Autodesk Inventor part; units mm, degrees
ref_plane "Work Plane1" through (0, -9.525, 0) normal (0, -1, 0) x (1, 0, 0)
ref_plane "Work Plane2" through (0, 9.525, 0) normal (0, 1, 0) x (1, 0, 0)
ref_plane "YZ Plane" through (0, 0, 0) normal (1, 0, 0) x (0, 1, 0)
sketch "Sketch1" plane through (0, 0, 0) normal (0, 0, 1) x (1, 0, 0)
  line L0 (-3.3274, -3.3274) -> (3.3274, -3.3274)
  line L1 (3.3274, -3.3274) -> (3.3274, 3.3274)
  line L2 (3.3274, 3.3274) -> (-3.3274, 3.3274)
  line L3 (-3.3274, 3.3274) -> (-3.3274, -3.3274)
  line L4 (-3.3274, -3.3274) -> (3.3274, 3.3274) construction
  line L5 (3.3274, -3.3274) -> (-3.3274, 3.3274) construction
  circle A0 centre (0, 0) radius 9.525
  line L6 (-4.5974, 0.3969) -> (11.7358, 0.3969)
  line L7 (11.7358, 0.3969) -> (11.7358, -0.3969)
  line L8 (11.7358, -0.3969) -> (-4.5974, -0.3969)
  line L9 (-4.5974, -0.3969) -> (-4.5974, 0.3969)
  point P0 (-4.5974, 0)
  point P1 (-3.3274, -0.3969)
  point P2 (-3.3274, 0.3969)
  point P3 (3.3274, 0.3969)
  point P4 (9.5167, 0.3969)
  point P5 (9.5167, -0.3969)
  point P6 (3.3274, -0.3969)
  dimension "d0" = 6.6548
  dimension "d1" = 6.6548
  dimension "d2" = 19.05
  dimension "d3" = 0.7937
  dimension "d4" = 1.27
extrude "Extrusion1" add sketch "Sketch1" along normal blind 63.5 contours L0 L1 L8 A0 L6 L2 L3 L9
sketch "Sketch2" plane through (3.3274, 0.3969, 0) normal (0, -1, 0) x (1, 0, 0)
  circle A0 centre (3.0947, 57.15) radius 2.286
  line L0 (0, 63.5) -> (6.1893, 63.5)
  line L1 (6.1893, 0) -> (6.1893, 63.5)
  line L2 (6.1893, 31.75) -> (0, 31.75)
  line L3 (0, 0) -> (0, 63.5)
  circle A1 centre (3.0947, 6.35) radius 2.286
  point P0 (-3.3274, 0)
  point P1 (3.0947, 63.5)
  dimension "d7" = 4.572
  dimension "d8" = 6.35
extrude "Extrusion2" cut sketch "Sketch2" along normal mid plane 63.5 contours A0 | A1
ref_plane "Work Plane1" through (0, -9.525, 0) normal (0, -1, 0) x (1, 0, 0)
ref_plane "Work Plane2" through (0, 9.525, 0) normal (0, 1, 0) x (1, 0, 0)
sketch "Sketch3" plane through (0, -9.525, 0) normal (0, -1, 0) x (1, 0, 0)
  circle A0 centre (6.4221, 6.35) radius 2.286
  circle A1 centre (6.4221, 6.35) radius 4.1275
  line L0 (6.4221, 10.4775) -> (9.5167, 10.4775)
  line L1 (9.5167, 0) -> (9.5167, 63.5)
  line L2 (6.4221, 2.2225) -> (9.5167, 2.2225)
  line L3 (-9.525, 0) -> (-9.525, 63.5)
  line L4 (-9.525, 31.75) -> (9.5167, 31.75)
  circle A2 centre (6.4221, 57.15) radius 4.1275
  line L5 (6.4221, 53.0225) -> (9.5167, 53.0225)
  line L6 (6.4221, 61.2775) -> (9.5167, 61.2775)
  point P0 (0, 0)
  dimension "d11" = 8.255
extrude "Extrusion3" cut sketch "Sketch3" against normal blind 5.715 contours A1 L1 | L0 L1 A1 | A1 L1 L2 | L5 A2 L1 | A2 L1 | A2 L6 L1 picked at (9.2472, 6.35) picked at (7.5728, 58.1798)
sketch "Sketch4" plane through (0, 9.525, 0) normal (0, 1, 0) x (1, 0, 0)
  circle A0 centre (6.4221, -6.35) radius 2.286
  arc A1 (6.4221, -2.2225) -> (6.4221, -10.4775) centre (6.4221, -6.35) ccw
  line L0 (0.9228, -6.35) -> (3.6724, -1.5875)
  line L1 (3.6724, -1.5875) -> (9.1717, -1.5875)
  line L2 (9.1717, -1.5875) -> (11.9213, -6.35)
  line L3 (11.9213, -6.35) -> (9.1717, -11.1125)
  line L4 (9.1717, -11.1125) -> (3.6724, -11.1125)
  line L5 (3.6724, -11.1125) -> (0.9228, -6.35)
  line L6 (-9.525, 0) -> (-9.525, -63.5)
  line L7 (-9.525, -31.75) -> (9.525, -31.75)
  line L8 (9.1717, -11.1125) -> (11.7374, -11.1125)
  line L9 (11.7374, -11.1125) -> (11.7374, -1.5875)
  line L10 (11.7374, -1.5875) -> (9.1717, -1.5875)
  line L11 (0.9228, -57.15) -> (3.6724, -61.9125)
  line L12 (3.6724, -61.9125) -> (9.1717, -61.9125)
  line L13 (9.1717, -61.9125) -> (11.9213, -57.15)
  line L14 (11.9213, -57.15) -> (9.1717, -52.3875)
  line L15 (9.1717, -52.3875) -> (3.6724, -52.3875)
  line L16 (3.6724, -52.3875) -> (0.9228, -57.15)
  line L17 (9.1717, -52.3875) -> (11.7374, -52.3875)
  line L18 (11.7374, -52.3875) -> (11.7374, -61.9125)
  line L19 (11.7374, -61.9125) -> (9.1717, -61.9125)
  point P0 (0, 0)
  point P1 (11.7374, -6.6685)
  point P2 (11.7374, -6.0315)
  dimension "d16" = 9.525
extrude "Extrusion4" cut sketch "Sketch4" against normal blind 6.096 contours A0 | L0 L1 L2 L9 L3 L4 L5 | L10 L9 L2 | L3 L9 L8 | L16 L15 L14 L18 L13 L12 L11 | L13 L18 L19 | L17 L18 L14
sketch "Sketch5" plane through (0, 0, 63.5) normal (0, 0, 1) x (1, 0, 0)
  line L0 (4.1361, -3.81) -> (8.7081, -3.81)
  arc A0 (9.5167, 0.3969) -> (9.5167, -0.3969) centre (0, 0) ccw
  line L1 (8.1359, -4.953) -> (-8.1359, -4.953)
  arc A1 (-8.1359, -4.953) -> (8.1359, -4.953) centre (0, 0) ccw
  dimension "d17" = 1.143
extrude "Extrusion5" cut sketch "Sketch5" against normal up to surface (63.5 mm away)
fillet "Fillet1" radius 3.175 1 edges at (-8.1359, -4.953, 31.75)
fillet "Fillet2" radius 2.54 3 edges at (8.1359, -4.953, 31.75) (8.1359, -4.953, 62.3888) (8.1359, -4.953, 1.1112)
properties part number "AxleBar"
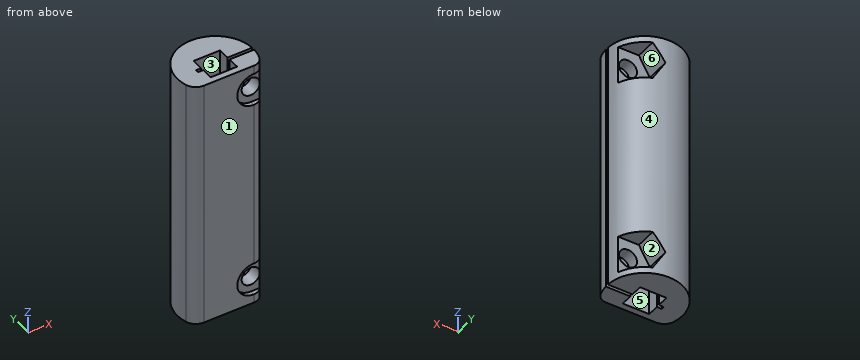
The listing builds one solid part. Answer for the finished solid, in the listing's coordinates (mm). Face numbers are marked on the shaded views. A direction names the side the tool comes from. Round coordinates to 2 decimals unless told otherwise and drop trailing zeros. Order: outer loops, then holes, each group sorted by start corner. A loop starts at its lowest first (then second) coordinate and runs counter-clockwise, first axis right, second up. Notation, with made-up numbers: (9.25, -18) -> (53.25, -18) arc R11 ccw to (53.25, -7) -> close; hole circle Ø5 at (3.25, 39). An arc over 180 degrees is marked (long way). One line per item, written item: value.
Item 1: For a pull along X with two mould halves and no side action, classify the marked faces 3, 4, 5 and 6 as released by +X, released by -X, zero draft, split by the parting line, or undercut.
Taken from the geometry:
face 3: undercut
face 4: split by the parting line
face 5: undercut
face 6: released by +X
Item 2: Find section A-A, the plane x = 0. Give the vertices of the cut face in (y, z) (3 decimals), then the cut area to 3 significant figures.
Taken from the geometry:
outline: (-4.953, 0) -> (-3.327, 0) -> (-3.327, 63.5) -> (-4.953, 63.5) -> close; (3.327, 0) -> (9.525, 0) -> (9.525, 63.5) -> (3.327, 63.5) -> close
area: 497 mm2
Item 3: For the marked faces 1 and 2, determine the directions among +Z, -Z, +X, -X, +Y, -Y from which every point of the face is accessible in a straight line to the end or side of a thin tool.
Taken from the geometry:
face 1: +Z, -Z, +X, -X, -Y
face 2: +X, +Y
Item 4: Straight lines are drawn through the part: L1, parallel to Z at x = 6.5, y = 5.25; L2, parallel to Z at x = 6.5, y = 2.5; L3, parallel to Y at x = 1, z = 20. For each, find the intervals that lie inside material, in ascending order.
Taken from the geometry:
L1: z = 0 to 1.59, 11.11 to 52.39, 61.91 to 63.5
L2: z = 0 to 4.07, 8.63 to 54.87, 59.43 to 63.5
L3: y = -4.95 to -3.33, 3.33 to 9.47
Item 5: Given P1, Ø3, axis at y = 5.5, z = 18, coming from the -X side; P2, Ø3, axis at x = -5, z = 44, coming from the +Y side; P3, Ø3, axis at x = 7, z = 44.5, coming from the +Y side; P4, Ø2.5, axis at x = 6.42, z = 57.15, coming from the +Y side, each flat-ended and moving along its own axis, determine where each tip first touches the part or whether it passes through.
Taken from the geometry:
P1: stops at x = -8.64
P2: stops at y = 8.86
P3: stops at y = 7.78
P4: passes through
Item 6: Find section C-C, the plane z = 12. Give the vertices of the cut face in (x, y) (3 decimals), then the cut area to 3 significant figures.
Taken from the geometry:
outline: (-9.144, -2.667) arc R3.175 ccw to (-6.096, -4.953) -> (6.555, -4.953) arc R2.54 ccw to (8.939, -3.29) arc R9.525 ccw to (9.517, -0.397) -> (3.327, -0.397) -> (3.327, -3.327) -> (-3.327, -3.327) -> (-3.327, -0.397) -> (-4.597, -0.397) -> (-4.597, 0.397) -> (-3.327, 0.397) -> (-3.327, 3.327) -> (3.327, 3.327) -> (3.327, 0.397) -> (9.517, 0.397) arc R9.525 ccw (long way) to start
area: 181 mm2
Item 7: Find section D-D, the plane y = 5.75. Give the vertices of the cut face in (x, z), then the cut area to 4 significant figures.
Taken from the geometry:
outline: (-7.59, 0) -> (7.59, 0) -> (7.59, 1.59) -> (3.67, 1.59) -> (0.92, 6.35) -> (3.67, 11.11) -> (7.59, 11.11) -> (7.59, 52.39) -> (3.67, 52.39) -> (0.92, 57.15) -> (3.67, 61.91) -> (7.59, 61.91) -> (7.59, 63.5) -> (-7.59, 63.5) -> close
area: 863.5 mm2
Item 8: Find section B-B, the plane y = 2. Give the vertices of the cut face in (x, z), then the cut area to 3 significant figures.
Taken from the geometry:
outline: (-9.31, 0) -> (-3.33, 0) -> (-3.33, 63.5) -> (-9.31, 63.5) -> close; (3.33, 0) -> (9.31, 0) -> (9.31, 63.5) -> (3.33, 63.5) -> close; hole circle Ø4.57 at (6.42, 6.35); hole circle Ø4.57 at (6.42, 57.15)
area: 727 mm2
